Part model, mm, in its own coordinate system. Face numbers are marked on the shaded views. A direction names the side the tool comes from. Give positions to 0.01 mm unless a question says otherwise; leave off trailing zeros. Write each loop counter-clockwise with the first axis right and the second up, starting at its lowest first coordinate (ties: lowest second). Pieces come first, ordered by that corner, then holes. Notation, with made-up numbers: (-26, -19.5) - (12, -19.5) arc R19 cw to (12, -3.5) - close; hole circle Ø5 at (-23.5, 75.25). An arc over 180 degrees is marked (long way). Answer as a JSON object with one key per item and string values. Group by question number.
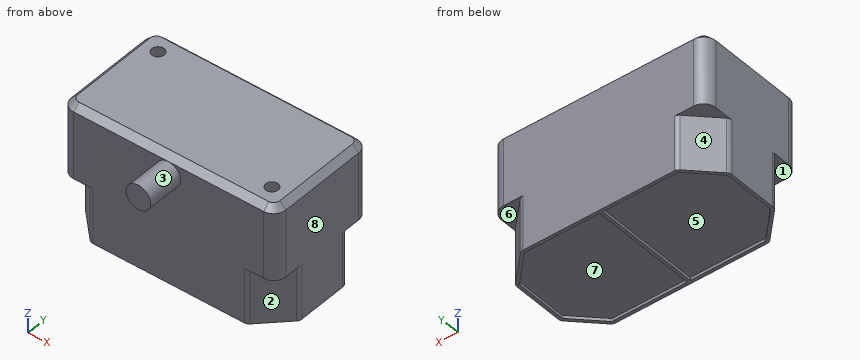
```python
from build123d import *

# Parameters (mm, degrees)
ESQUISSE1_W             = 35
ESQUISSE1_H             = 18.5
BOSS_EXTRU_1_DEPTH      = 21
CONG_1_R                = 2
ESQUISSE2_R             = 1
ENL_V_MAT_EXTRU_1_DEPTH = 4
ESQUISSE3_OUTSIDE_W     = 45.962
ESQUISSE3_OUTSIDE_H     = 29.462
ENL_V_MAT_EXTRU_2_DEPTH = 9
CONG_2_R                = 1
ENL_V_MAT_EXTRU_3_DEPTH = 0.5
ESQUISSE5_R             = 2
BOSS_EXTRU_2_DEPTH      = 6
CHANFREIN1_SIZE         = 1


with BuildPart() as part:
    # Esquisse1 → Boss.-Extru.1 (new body)
    with BuildSketch(Plane.XY):
        Rectangle(ESQUISSE1_W, ESQUISSE1_H)
    extrude(amount=BOSS_EXTRU_1_DEPTH)

    # Congé1
    cong_1_edges = [part.edges().sort_by_distance(p)[0] for p in [
        (-17.5, 9.25, 10.5),
        (17.5, 9.25, 10.5),
        (17.5, -9.25, 10.5),
        (-17.5, -9.25, 10.5),
    ]]
    fillet(cong_1_edges, radius=CONG_1_R)

    # Esquisse2 → Enlèv. mat.-Extru.1 (cut)
    with BuildSketch(Plane.XY.offset(21)):
        with Locations((-14, 5.75)):
            Circle(ESQUISSE2_R)
        with Locations((14, -5.75)):
            Circle(ESQUISSE2_R)
    extrude(amount=-ENL_V_MAT_EXTRU_1_DEPTH, mode=Mode.SUBTRACT)

    # Esquisse3 outside → Enlèv. mat.-Extru.2 (cut)
    with BuildSketch(Plane(origin=(0, 0, 0), x_dir=(-1, 0, 0), z_dir=(0, 0, -1))):
        Rectangle(ESQUISSE3_OUTSIDE_W, ESQUISSE3_OUTSIDE_H)
        Polygon((-17.5, 4.5), (-12.75, 9.25), (12.75, 9.25), (17.5, 4.5), (17.5, -4.5), (12.75, -9.25), (-12.75, -9.25), (-17.5, -4.5), align=None, mode=Mode.SUBTRACT)
    extrude(amount=-ENL_V_MAT_EXTRU_2_DEPTH, mode=Mode.SUBTRACT)

    # Congé2
    cong_2_edges = [part.edges().sort_by_distance(p)[0] for p in [
        (17.5, 4.5, 4.5),
        (12.75, 9.25, 4.5),
        (-12.75, 9.25, 4.5),
        (-17.5, 4.5, 4.5),
        (-17.5, -4.5, 4.5),
        (-12.75, -9.25, 4.5),
        (12.75, -9.25, 4.5),
        (17.5, -4.5, 4.5),
    ]]
    fillet(cong_2_edges, radius=CONG_2_R)

    # Esquisse4 → Enlèv. mat.-Extru.3 (cut)
    with BuildSketch(Plane(origin=(0, 0, 0), x_dir=(-1, 0, 0), z_dir=(0, 0, -1))):
        with BuildLine():
            Line((-0.25, 8.75), (-0.25, -8.75))
            Line((-0.25, -8.75), (-12.335786438, -8.75))
            ThreePointArc((-12.335786438, -8.75), (-12.527128154, -8.711939766), (-12.689339828, -8.603553391))
            Line((-12.689339828, -8.603553391), (-16.853553391, -4.439339828))
            ThreePointArc((-16.853553391, -4.439339828), (-16.961939766, -4.277128154), (-17, -4.085786438))
            Line((-17, -4.085786438), (-17, 4.085786438))
            ThreePointArc((-17, 4.085786438), (-16.961939766, 4.277128154), (-16.853553391, 4.439339828))
            Line((-16.853553391, 4.439339828), (-12.689339828, 8.603553391))
            ThreePointArc((-12.689339828, 8.603553391), (-12.527128154, 8.711939766), (-12.335786438, 8.75))
            Line((-12.335786438, 8.75), (-0.25, 8.75))
        make_face()
        with BuildLine():
            Line((0.25, 8.75), (0.25, -8.75))
            Line((0.25, -8.75), (12.335786438, -8.75))
            ThreePointArc((12.335786438, -8.75), (12.527128154, -8.711939766), (12.689339828, -8.603553391))
            Line((12.689339828, -8.603553391), (16.853553391, -4.439339828))
            ThreePointArc((16.853553391, -4.439339828), (16.961939766, -4.277128154), (17, -4.085786438))
            Line((17, -4.085786438), (17, 4.085786438))
            ThreePointArc((17, 4.085786438), (16.961939766, 4.277128154), (16.853553391, 4.439339828))
            Line((16.853553391, 4.439339828), (12.689339828, 8.603553391))
            ThreePointArc((12.689339828, 8.603553391), (12.527128154, 8.711939766), (12.335786438, 8.75))
            Line((12.335786438, 8.75), (0.25, 8.75))
        make_face()
    extrude(amount=-ENL_V_MAT_EXTRU_3_DEPTH, mode=Mode.SUBTRACT)

    # Esquisse5 → Boss.-Extru.2 (add)
    with BuildSketch(Plane.XZ.offset(9.25)):
        with Locations(Location((-0.035714286, 18, 0), (0, 0, 180))):
            Circle(ESQUISSE5_R)
    extrude(amount=BOSS_EXTRU_2_DEPTH)

    # Chanfrein1
    chanfrein1_edges = [part.edges().sort_by_distance(p)[0] for p in [
        (0, -9.25, 21),
        (-17.5, 0, 21),
        (17.5, 0, 21),
        (0, 9.25, 21),
        (16.914213562, 8.664213562, 21),
        (-16.914213562, 8.664213562, 21),
        (16.914213562, -8.664213562, 21),
        (-16.914213562, -8.664213562, 21),
    ]]
    chamfer(chanfrein1_edges, length=CHANFREIN1_SIZE - 0.0001)  # a hair under: the kernel refuses the full size


solid = part.part
```
1) Mould opens along X. For the marked faces 6, 7 and 8 say: pulls with the +X half, pulls with the -X half, needs draft (parallel to the pull), parting line crosses it, or undercut.
2) Band-saw the part on A-A (z = 18). List the corners of the cut face in (x, y), plus the area to 3 significant figures.
3) Band-saw the part on C-C (y = -2.5). List the corners of the cut face in (x, z), plus the area to 3 significant figures.
4) Band-saw the part on D-D (z = 5.75). List the corners of the cut face in (x, y), plus the area to 3 significant figures.
5) Band-saw the part on B-B (x = 3.5). List the corners of the cut face in (y, z).
6) Which spindle directions (+Z, -Z, +X, -X, +Y, -Y) get a long thin tool onto all of the face, cutting with end or side? Do the marked faces 1, 2, 3, 4 and 5. Say none if no direction does.
7) Drop flat-ended pins along their axis: P1, Ø5, axis at x = 3, y = 3.5, coming from the -Z side; P2, Ø8, axis at x = -8.5, z = 17, coming from the -Y side; P3, Ø1.5, axis at x = 2.5, z = 10, coming from the -Y side. Give the stop position or say it passes through.
8) Probe line 1 (Y direction, x = 14, z = 18.25); line 2 (Y direction, x = -14, z = 18.8); line 3 (Z direction, x = 4, y = -0.5). List the from-to ranges inside material, lowest first.
Verdict:
{
 "1": {"face 6": "needs draft", "face 7": "undercut", "face 8": "pulls with the +X half"},
 "2": {"outline": "(-17.5, -7.25) arc R2 ccw to (-15.5, -9.25) - (-2.04, -9.25) - (-2.04, -15.25) - (1.96, -15.25) - (1.96, -9.25) - (15.5, -9.25) arc R2 ccw to (17.5, -7.25) - (17.5, 7.25) arc R2 ccw to (15.5, 9.25) - (-15.5, 9.25) arc R2 ccw to (-17.5, 7.25) - close; hole circle Ø2 at (-14, 5.75); hole circle Ø2 at (14, -5.75)", "area": "662 mm2"},
 "3": {"outline": "(-17.5, 0) - (-17, 0) - (-17, 0.5) - (-0.25, 0.5) - (-0.25, 0) - (0.25, 0) - (0.25, 0.5) - (17, 0.5) - (17, 0) - (17.5, 0) - (17.5, 20) - (16.5, 21) - (-16.5, 21) - (-17.5, 20) - close", "area": "717 mm2"},
 "4": {"outline": "(-17.5, -4.09) arc R1 ccw to (-17.21, -4.79) - (-13.04, -8.96) arc R1 ccw to (-12.34, -9.25) - (12.34, -9.25) arc R1 ccw to (13.04, -8.96) - (17.21, -4.79) arc R1 ccw to (17.5, -4.09) - (17.5, 4.09) arc R1 ccw to (17.21, 4.79) - (13.04, 8.96) arc R1 ccw to (12.34, 9.25) - (-12.34, 9.25) arc R1 ccw to (-13.04, 8.96) - (-17.21, 4.79) arc R1 ccw to (-17.5, 4.09) - close", "area": "602 mm2"},
 "5": {"outline": "(-9.25, 0) - (-8.75, 0) - (-8.75, 0.5) - (8.75, 0.5) - (8.75, 0) - (9.25, 0) - (9.25, 20) - (8.25, 21) - (-8.25, 21) - (-9.25, 20) - close"},
 "6": {"face 1": "-Z, -X, -Y", "face 2": "-Z, +X, -Y", "face 3": "-Y", "face 4": "-Z, -X, +Y", "face 5": "-Z"},
 "7": {"P1": "z = 0.5", "P2": "y = -9.25", "P3": "y = -9.25"},
 "8": {"line 1": "-9.25 to -6.75, -4.75 to 9.25", "line 2": "-9.25 to 4.75, 6.75 to 9.25", "line 3": "0.5 to 21"}
}
